Autodesk Inventor part; units mm, degrees
ref_plane "YZ Plane" through (0, 0, 0) normal (1, 0, 0) x (0, 1, 0)
ref_plane "XZ Plane" through (0, 0, 0) normal (0, 1, 0) x (-1, 0, 0)
ref_plane "XY Plane" through (0, 0, 0) normal (0, 0, 1) x (1, 0, 0)
sketch "Sketch1" plane through (0, 0, 0) normal (0, 1, 0) x (-1, 0, 0)
  line L0 (75, -60) -> (-75, -60)
  line L1 (-75, -60) -> (-75, 60)
  line L2 (-75, 60) -> (75, 60)
  line L3 (75, 60) -> (75, -60)
  line L4 (75, -60) -> (-75, 60) construction
  line L5 (-75, -60) -> (75, 60) construction
  point P0 (0, 0)
  dimension "d0" = 120
  dimension "d1" = 150
extrude "Extrusion1" add sketch "Sketch1" along normal blind 40
sketch "Sketch2" plane through (75, 0, 60) normal (1, 0, 0) x (0, 0, -1)
  line L0 (60, 0) -> (60, 40)
  line L1 (110, 35) -> (10, 35)
  line L2 (10, 35) -> (10, 5)
  line L3 (10, 5) -> (110, 5)
  line L4 (110, 5) -> (110, 35)
  line L5 (110, 35) -> (10, 5) construction
  line L6 (10, 35) -> (110, 5) construction
  line L7 (0, 40) -> (120, 40)
  point P0 (60, 20)
  dimension "d4" = 100
  dimension "d5" = 30
  dimension "d6" = 5
extrude "Extrusion2" cut sketch "Sketch2" against normal through all
sketch "Sketch3" plane through (75, 0, 60) normal (1, 0, 0) x (0, 0, -1)
  line L0 (60, 0) -> (60, 5)
  line L1 (110, 5) -> (10, 5)
  line L2 (100, 10) -> (20, 10)
  line L3 (20, 10) -> (20, -5)
  line L4 (20, -5) -> (100, -5)
  line L5 (100, -5) -> (100, 10)
  line L6 (100, 10) -> (20, -5) construction
  line L7 (20, 10) -> (100, -5) construction
  point P0 (60, 2.5)
  point P1 (100, 5)
  point P2 (20, 5)
  point P3 (110, 5)
  point P4 (0, 5)
  point P5 (100, 15)
  dimension "d9" = 80
extrude "Extrusion3" cut sketch "Sketch3" against normal through all
sketch "Sketch4" plane through (0, 40, 0) normal (0, 1, 0) x (1, 0, 0)
  line L0 (-50, 25) -> (50, 25)
  line L1 (50, 25) -> (50, -25)
  line L2 (50, -25) -> (-50, -25)
  line L3 (-50, -25) -> (-50, 25)
  line L4 (-50, 25) -> (50, -25) construction
  line L5 (50, 25) -> (-50, -25) construction
  point P0 (0, 0)
  dimension "d12" = 50
  dimension "d13" = 100
extrude "Extrusion4" cut sketch "Sketch4" against normal blind 3
sketch "Sketch5" plane through (75, 0, -60) normal (0, 0, -1) x (-1, 0, 0)
  line L0 (0, 0) -> (150, 0)
  line L1 (150, 0) -> (150, 40)
  line L2 (0, 40) -> (150, 40)
  line L3 (0, 0) -> (0, 40)
  line L4 (150, 0) -> (0, 0) construction
  line L5 (150, 0) -> (0, 40) construction
  line L6 (0, 0) -> (0, 40) construction
  line L7 (0, 0) -> (150, 40) construction
  line L8 (75, 20) -> (75, 40) construction
  line L9 (0, 40) -> (40, 40)
  line L10 (40, 0) -> (0, 0)
  line L11 (0, 0) -> (0, 40)
  line L12 (150, 0) -> (150, 40)
  line L13 (0, 30) -> (40, 30)
  line L14 (40, 30) -> (40, 0)
  line L15 (40, 0) -> (0, 0)
  line L16 (0, 0) -> (0, 30)
  line L17 (0, 30) -> (40, 0)
  line L18 (150, 30) -> (110, 30)
  line L19 (110, 30) -> (110, 0)
  line L20 (150, 30) -> (110, 0)
  point P0 (75, 0)
  point P1 (150, 30)
  point P2 (110, 0)
  point P3 (110, 0)
  dimension "d20" = 30
  dimension "d21" = 70
extrude "Extrusion5" cut sketch "Sketch5" against normal through all contours L3 L17 L0 | L20 L1 L0
sketch "Sketch6" plane through (-75, 40, 60) normal (0, 0, 1) x (1, 0, 0)
  line L0 (0, 0) -> (150, 0)
  line L1 (150, -10) -> (150, 0)
  line L2 (0, 0) -> (150, 0)
  line L3 (0, -10) -> (0, 0)
  line L4 (0, -10) -> (40, -40)
  line L5 (33.3333, -35) -> (116.6667, -35)
  line L6 (40, -40) -> (0, -10)
  line L7 (16, -22) -> (134, -22)
  line L8 (150, -10) -> (110, -40)
  line L9 (53, -22) -> (53, -35)
  line L10 (150, -35) -> (33.3333, -35)
  line L11 (75, -40) -> (75, 0)
  line L12 (25, 0) -> (125, 0) construction
  line L13 (97, -22) -> (97, -35)
  line L14 (0, -10) -> (40, -40)
  line L15 (40, -40) -> (110, -40)
  line L16 (110, -40) -> (150, -10)
  point P0 (97, -22)
  point P1 (97, -35)
  point P2 (16, -22)
  dimension "d22" = 13
  dimension "d24" = 22
extrude "Extrusion6" cut sketch "Sketch6" against normal through all contours L7 L9 L5 L4 | L7 L8 L5 L13
fillet "Fillet1" radius 5 4 edges at (22, 11.5, 50) (-22, 11.5, 50) (-22, 11.5, -50) (22, 11.5, -50)
fillet "Fillet2" radius 10 4 edges at (38.3333, 2.5, 40) (-38.3333, 2.5, 40) (-38.3333, 2.5, -40) (38.3333, 2.5, -40)
properties part number "Battery Cage"
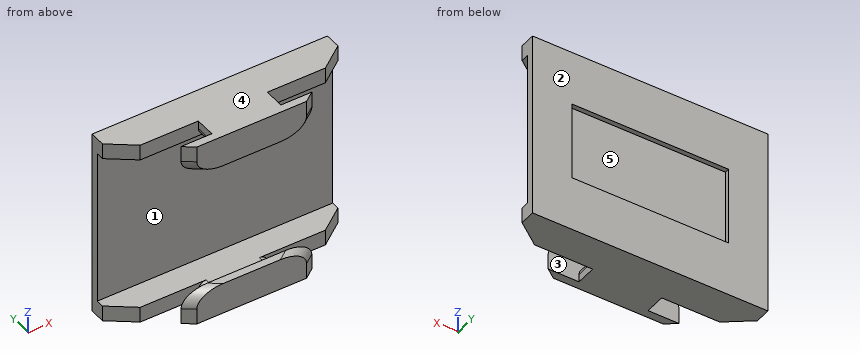
Model file for the job. Use its own axes, mm. Face numbers are marked on the shaded views. A direction names the side the tool comes from. Round coordinates to 2 decimals unless told otherwise and drop trailing zeros. Write each loop counter-clockwise with the first axis right and the second up, starting at its lowest first coordinate (ties: lowest second). Pieces come first, ordered by that corner, then holes. Notation, with made-up numbers: (-33, 51) - (3, 51) arc R30 ccw to (3, 76) - close; hole circle Ø11 at (-31, -19.5). An arc over 180 degrees is marked (long way). One line per item, written item: value.
(1) 3-axis set-ups, long thin cutter, end or side, ignore diameter. For the marked faces 1, 2 and 3: which of +Z, -Z, +X, -X, +Y, -Y reach the whole face in a straight line?
Values follow:
face 1: +X, -X
face 2: +Z, -Z, +X, -X, +Y
face 3: none
(2) Cut at D-D, the plane z = 44. Give the cut face in (x, y), plus the area to 3 significant figures.
Values follow:
outline: (-75, 35) - (75, 35) - (75, 40) - (-75, 40) - close; (-38.33, 5) - (-31.67, 0) - (31.67, 0) - (38.33, 5) - close
area: 1,100 mm²
(3) Wall check: probe 1 along Z at (x, y) = (-66, 27.5); probe 2 along Y at (x, z) = (-3.5, -41.5); probe 3 along Y at (x, z) = (-47, 12). Give the ranges that are in metal, low to high.
Values follow:
probe 1: z = -60 to -50, 50 to 60
probe 2: y = 0 to 5, 35 to 40
probe 3: y = 35 to 37
(4) Cut at B-B, the plane z = 4.5. Give the cut face in (x, y).
Values follow:
outline: (-75, 35) - (75, 35) - (75, 40) - (50, 40) - (50, 37) - (-50, 37) - (-50, 40) - (-75, 40) - close
(5) Cut at A-A, the plane y = 33. Give the cut face in (x, z).
Values follow:
outline: (-75, -60) - (75, -60) - (75, -50) - (-75, -50) - close; (-75, 50) - (75, 50) - (75, 60) - (-75, 60) - close
(6) Drop flat-ended pins along their axis: P1, Ø5.5, axis at y = 13, z = 58, coming from the +X side; P2, Ø11, axis at x = -46, z = -54, coming from the -Y side (3 decimals); P3, Ø4, axis at x = -45.5, z = -7.5, coming from the -Y side; P4, Ø8, axis at x = -34.5, z = 53, coming from the -Y side. Give the stop position or say it passes through.
Values follow:
P1: stops at x = 22
P2: stops at y = 4.125
P3: stops at y = 35
P4: stops at y = 0
(7) Cut at C-C, the plane x = 8.5. Give the cut face in (y, z).
Values follow:
outline: (0, -60) - (40, -60) - (40, -25) - (37, -25) - (37, 25) - (40, 25) - (40, 60) - (0, 60) - (0, 40) - (5, 40) - (5, 50) - (35, 50) - (35, -50) - (5, -50) - (5, -40) - (0, -40) - close
(8) Two-plate mould, pull along X, no slides. Class the marked faces 4 and 5: pulls with the +X half, pulls with the -X half, needs draft (parallel to the pull), parting line crosses it, or undercut.
Values follow:
face 4: needs draft
face 5: undercut
